```python
from build123d import *

# Parameters (mm, degrees)
REVOLVE1_ANGLE      = 180
SHELL2_T            = -1.2
SKETCH4_W           = 16.30613237
SKETCH4_H           = 1.2
SKETCH4_W_2         = 16.004639453
SKETCH4_W_3         = 1.2
SKETCH4_H_2         = 16.004639453
BOSS_EXTRUDE1_DEPTH = 1
SKETCH5_W           = 1.2
SKETCH5_H           = 1
SKETCH5_W_2         = 1
SKETCH5_H_2         = 1.2
BOSS_EXTRUDE2_DEPTH = 5


with BuildPart() as part:
    # Sketch3 → Revolve1 (revolve)
    with BuildSketch(Plane(origin=(0, 0, 0), x_dir=(1, 0, 0), z_dir=(0, 1, 0))):
        with BuildLine():
            Line((-40, 0), (40, 0))
            ThreePointArc((40, 0), (0, 40), (-40, 0))
        make_face()
    revolve(axis=Axis((-40, 0, 0), (1, 0, 0)), revolution_arc=REVOLVE1_ANGLE)

    # Shell2
    shell2_openings = [part.faces().sort_by_distance(p)[0] for p in [
        (0, 0, 0),
    ]]
    offset(amount=SHELL2_T, openings=shell2_openings)

    # Sketch4 → Boss-Extrude1 (add)
    with BuildSketch(Plane.XZ):
        with Locations((-31.248426732, 0)):
            Rectangle(SKETCH4_W, SKETCH4_H)
        with Locations((31.097680274, 0)):
            Rectangle(SKETCH4_W_2, SKETCH4_H)
        with Locations((0, -31.097680274)):
            Rectangle(SKETCH4_W_3, SKETCH4_H_2)
        with Locations((0, 31.097680274)):
            Rectangle(SKETCH4_W_3, SKETCH4_H_2)
    extrude(amount=-BOSS_EXTRUDE1_DEPTH)

    # Sketch5 → Boss-Extrude2 (add)
    with BuildSketch(Plane.XZ):
        with Locations((0, 23.595360547)):
            Rectangle(SKETCH5_W, SKETCH5_H)
        with Locations((-23.595360547, 0)):
            Rectangle(SKETCH5_W_2, SKETCH5_H_2)
        with Locations((23.595360547, 0)):
            Rectangle(SKETCH5_W_2, SKETCH5_H_2)
        with Locations((0, -23.595360547)):
            Rectangle(SKETCH5_W, SKETCH5_H)
    extrude(amount=BOSS_EXTRUDE2_DEPTH)


solid = part.part
```
Geometry: final body of the model. Coordinates: model frame, mm. Round coordinates to 2 decimals unless told otherwise and drop trailing zeros. Order: outer loops, then holes, each group sorted by start corner. A loop starts at its lowest first (then second) coordinate and runs counter-clockwise, first axis right, second up. Notation, with made-up numbers: (8, 89) -> (51, 89) arc R8 ccw to (51, 99) -> close; hole circle Ø4 at (8.5, 17.5). An arc over 180 degrees is marked (long way). Use one line per item in the form item = value. Start each with the question number.
1. Cut plane C-C (y = 37.5). Return the cut outline in (x, z).
2. Cut plane A-A (z = -30). Return the cut outline in (x, y), then the cut area to 3 significant figures.
3. Cut plane B-B (x = 30.5). Return the cut outline in (y, z), then the cut area to 3 significant figures.
4. Cut plane D-D (z = 21.5). Return the cut outline in (x, y).
5. Pin query (flat end, axial travel): pin 1 Ø1.3 at (x, y) = (0, -2) entering from +Z; pin 2 Ø10 at (x, y) = (-16, 14) entering from -Z; pin 3 Ø2 at (x, z) = (-3, -17) entering from -Y. Return the tip coordinate at first contact, or that it passes through.
6. Line query: probe 1 along X at (y, z) = (1, 12); probe 2 along X at (y, z) = (6, 21); probe 3 along Z at (x, y) = (0, 29.5). Output: solid intervals per line, ascending.
7. Draft query along Z for faces 1 (the face through (-0.6, 0.2, -29.2)), 2 (the face through (-27, 0, 0)). Return one class per face: pulls with the +Z half, pulls with the -Z half, needs draft (parallel to the pull), parting line crosses it, or undercut.
Solution:
q1.outline = circle Ø27.84 at (0, 0); hole circle Ø19.92 at (0, 0)
q2.outline = (-26.46, 0) -> (-24.61, 0) arc R24.61 cw to (24.61, 0) -> (26.46, 0) arc R26.46 ccw to start; (-0.6, 0) -> (0.6, 0) -> (0.6, 1) -> (-0.6, 1) -> close
q2.area = 150 mm^2
q3.outline = (0, -25.88) arc R25.88 ccw to (0, 25.88) -> (0, 23.98) arc R23.98 cw to (0, -23.98) -> close; (0, -0.6) -> (1, -0.6) -> (1, 0.6) -> (0, 0.6) -> close
q3.area = 150 mm^2
q4.outline = (-33.73, 0) -> (-32.3, 0) arc R32.3 cw to (32.3, 0) -> (33.73, 0) arc R33.73 ccw to start
q5.pin_1 = 24.1
q5.pin_2 = -36.55
q5.pin_3 = 34.23
q6.probe_1 = -38.14 to -36.88, 36.88 to 38.14
q6.probe_2 = -33.51 to -32.07, 32.07 to 33.51
q6.probe_3 = -27.01 to -25.2, 25.2 to 27.01
q7.face_1 = undercut
q7.face_2 = needs draft
